```python
from build123d import *

# Parameters (mm, degrees)
SKETCH2_W          = 28
SKETCH2_H          = 5.2
CUT_EXTRUDE1_DEPTH = 40


with BuildPart() as part:
    # Sketch1 → Revolve1 (revolve)
    with BuildSketch(Plane(origin=(0, 0, 0), x_dir=(1, 0, 0), z_dir=(0, 1, 0))):
        Polygon((0, 0), (-1040, 0), (-1040, 50), (-950, 50), (-950, 137), (0, 137), (950, 137), (950, 50), (1180, 50), (1180, 0), align=None)
    revolve(axis=Axis((0, 0, 0), (-1, 0, 0)))

    # Sketch2 → Cut-Extrude1 (cut)
    with BuildSketch(Plane(origin=(1180, 0, 0), x_dir=(0, 0, -1), z_dir=(1, 0, 0))):
        with Locations((0, 48)):
            Rectangle(SKETCH2_W, SKETCH2_H)
    extrude(amount=-CUT_EXTRUDE1_DEPTH, mode=Mode.SUBTRACT)


solid = part.part
```
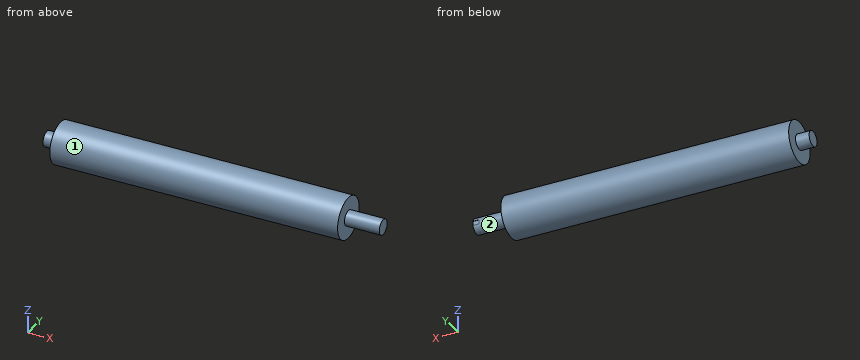
Geometry check sheet. Reference: the model listing, model coordinates, mm. Face numbers are marked on the shaded views. A direction names the side the tool comes from. Round coordinates to 2 decimals unless told otherwise and drop trailing zeros. Write each loop counter-clockwise with the first axis right and the second up, starting at its lowest first coordinate (ties: lowest second). Pieces come first, ordered by that corner, then holes. Notation, with made-up numbers: (11.25, 70.25) -> (43.25, 70.25) arc R27 cw to (43.25, 86.25) -> close; hole circle Ø9 at (76, -7). An arc over 180 degrees is marked (long way). Put each result on its own line as item: value.
1) Cross-section at D-D, the plane x = 1027.5. Enter the section's corners in (y, z), plus the area to 3 significant figures.
Recorded:
outline: circle Ø100 at (0, 0)
area: 7,850 mm2
2) Cross-section at A-A, the plane y = 0. Enter the section's corners in (x, z).
Recorded:
outline: (-1040, -50) -> (-950, -50) -> (-950, -137) -> (950, -137) -> (950, -50) -> (1180, -50) -> (1180, 50) -> (950, 50) -> (950, 137) -> (-950, 137) -> (-950, 50) -> (-1040, 50) -> close
3) Access from +Z, -Z, +X, -X, +Y, -Y to the whole of each face (thin tool, end or side, straight path). Record for the marked faces 1 and 2.
Recorded:
face 1: +X, -X
face 2: +X
4) Cross-section at C-C, the plane z = 118.5. Enter the section's corners in (x, y).
Recorded:
outline: (-950, -68.75) -> (950, -68.75) -> (950, 68.75) -> (-950, 68.75) -> close
5) Depth check by flat-ended pin: P1, Ø12, axis at x = -424, z = 68.5, coming from the -Y side; P2, Ø12, axis at x = 159.5, y = -38.5, coming from the +Z side; P3, Ø4, axis at x = 369.5, z = -45.5, coming from the +Y side. Enter the tip coordinate at first touch or a pass-through.
Recorded:
P1: stops at y = -121.91
P2: stops at z = 133.09
P3: stops at y = 129.91
6) Cross-section at B-B, the plane x = -308.5. Enter the section's corners in (y, z), plus the area to 3 significant figures.
Recorded:
outline: circle Ø274 at (0, 0)
area: 59,000 mm2
7) Thickness scan on probe 1 along X at (y, z) = (28.5, -122); probe 2 along Y at (x, z) = (375.5, -5); probe 3 along Y at (x, z) = (278, 2). Record the ranges inside material, lowest first. Write a range as from..to.
Recorded:
probe 1: x = -950..950
probe 2: y = -136.91..136.91
probe 3: y = -136.99..136.99
